Source: CAD feature listing. Evaluate the final solid. Frame: model axes, mm. Face numbers are marked on the shaded views. A direction names the side the tool comes from. Round coordinates to 2 decimals unless told otherwise and drop trailing zeros. Write each loop counter-clockwise with the first axis right and the second up, starting at its lowest first coordinate (ties: lowest second). Pieces come first, ordered by that corner, then holes.
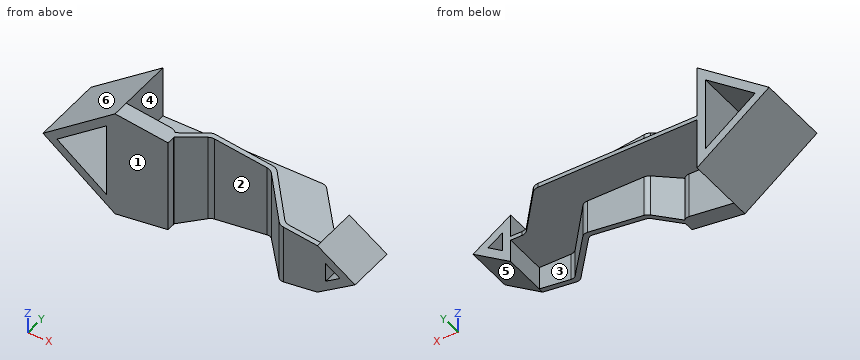
```python
from build123d import *

# Parameters (mm, degrees)
EXTRUDE_1_DEPTH             = 86
EXTRUDE_1_2_DEPTH           = 64.5
EXTRUDE_1_2_DEPTH_BACK      = 64.5
EXTRUDE_5_DEPTH             = 57.333333333
CUT_EXTRUDE_5_DEPTH         = 328.099755426
CUT_EXTRUDE_5_DEPTH_BACK    = 328.099755426
SKETCH_13_OUTSIDE_W         = 475.92
SKETCH_13_OUTSIDE_H         = 215.92
RIB_START                   = -2.5
RIB_2_DEPTH                 = 5
FILLET_1_R                  = 10
CUT_EXTRUDE_3_DEPTH         = 322.504665596
CUT_EXTRUDE_3_DEPTH_BACK    = 322.504665596
SKETCH_10_R                 = 5
CUT_EXTRUDE_4_DEPTH         = 322.504665596
CUT_EXTRUDE_4_DEPTH_BACK    = 322.504665596
SKETCH_11_R                 = 5
EXTRUDE_6_REACH             = 323.505
EXTRUDE_6_DIRECTION_2_REACH = 323.505


# Read off the part's stored shape, not the designer's step: 보강대2
with BuildPart() as part:
    # 스케치1 → Extrude 1 (new body)
    with BuildSketch(Plane(origin=(0, 0, 0), x_dir=(1, 0, 0), z_dir=(0, 1, 0))):
        Polygon((0, 64.5), (0, -64.5), (-86, 0), align=None)
        Polygon((-10, 44.5), (-69.333333333, 0), (-10, -44.5), align=None, mode=Mode.SUBTRACT)
    extrude(amount=EXTRUDE_1_DEPTH)


with BuildPart() as body_2:
    # 스케치3 → Extrude 1 2 (new, two sides: drawn at the far end of the back side and taken through both)
    with BuildSketch(Plane.XY.offset(-EXTRUDE_1_2_DEPTH_BACK)):
        Polygon((0, 0), (50, 0), (91.711375741, 35), (162.654022129, 35), (213, -25), (258, -25), (258, -19), (215.797845949, -19), (165.451868078, 41), (89.527554335, 41), (47.816178594, 6), (0, 6), align=None)
    extrude(amount=EXTRUDE_1_2_DEPTH + EXTRUDE_1_2_DEPTH_BACK)

    # 스케치13 outside → 컷-돌출5 (cut, two sides: drawn at the far end of the back side and taken through both)
    with BuildSketch(Plane(origin=(0, -19, 0), x_dir=(1, 0, 0), z_dir=(0, 1, 0)).offset(-CUT_EXTRUDE_5_DEPTH_BACK)):
        with Locations((108.5, 0)):
            Rectangle(SKETCH_13_OUTSIDE_W, SKETCH_13_OUTSIDE_H)
        Polygon((0, 64.5), (258, 30), (258, -30), (0, -64.5), align=None, mode=Mode.SUBTRACT)
    extrude(amount=CUT_EXTRUDE_5_DEPTH + CUT_EXTRUDE_5_DEPTH_BACK, mode=Mode.SUBTRACT)


with BuildPart() as body_3:
    # 스케치12 → 보스-돌출5 (new body)
    with BuildSketch(Plane.XZ.offset(25)):
        Polygon((258, 30), (258, -30), (303, 0), align=None)
        Polygon((268, 11.314829082), (284.972243623, 0), (268, -11.314829082), align=None, mode=Mode.SUBTRACT)
    extrude(amount=-EXTRUDE_5_DEPTH)


with BuildPart() as part_1:
    add(part.part)

    # Combine 1: union body 3, body 2
    add(body_3.part)
    add(body_2.part)

    # 보강대2 outline → 보강대2 (add)
    with BuildSketch(Plane.XY.offset(RIB_START)):
        Polygon((239.734972401, 32.333333333), (194.703292194, 86), (0, 86), (0, 6), (47.816178594, 6), (89.527554335, 41), (165.451868078, 41), (215.797845949, -19), (258, -19), (258, 32.333333333), align=None)
    extrude(amount=RIB_2_DEPTH)

    # 필렛1
    fillet_1_edges = [part_1.edges().sort_by_distance(p)[0] for p in [
        (194.703292194, 86, 0),
        (213, -25, 0),
        (215.797845949, -19, 19.071655649),
        (165.451868078, 41, 22.437811146),
        (89.527554335, 41, 27.514146076),
        (47.816178594, 6, 30.302988059),
        (50, 0, 0),
        (91.711375741, 35, 0),
        (162.654022129, 35, 0),
        (47.816178594, 6, -30.302988059),
        (89.527554335, 41, -27.514146076),
        (165.451868078, 41, -22.437811146),
        (215.797845949, -19, -19.071655649),
        (239.734972401, 32.333333333, 0),
    ]]
    fillet(fillet_1_edges, radius=FILLET_1_R)

    # 스케치10 → 컷-돌출3 (cut, two sides: drawn at the far end of the back side and taken through both)
    with BuildSketch(Plane.XY.offset(-CUT_EXTRUDE_3_DEPTH_BACK)):
        with Locations((158, -20)):
            Circle(SKETCH_10_R)
    extrude(amount=CUT_EXTRUDE_3_DEPTH + CUT_EXTRUDE_3_DEPTH_BACK, mode=Mode.SUBTRACT)

    # 스케치11 → 컷-돌출4 (cut, two sides: drawn at the far end of the back side and taken through both)
    with BuildSketch(Plane.XY.offset(-CUT_EXTRUDE_4_DEPTH_BACK)):
        with Locations(Location((53.25, 10, 0), (0, 0, 44.917604926))):
            Circle(SKETCH_11_R)
    extrude(amount=CUT_EXTRUDE_4_DEPTH + CUT_EXTRUDE_4_DEPTH_BACK, mode=Mode.SUBTRACT)

    # 보스-돌출6: up to this plane
    extrude_6_end = Plane(origin=(258, -25, 30), z_dir=(0.13254117731278448, 0, 0.9911774999043013))
    # 스케치8 → 보스-돌출6 (add, up to the surface)
    with BuildSketch(Plane.XY, mode=Mode.PRIVATE) as extrude_6_sk1:
        with BuildLine():
            Line((63.25, 0), (0, 0))
            Line((0, 0), (0, 20))
            Line((0, 20), (53.25, 20))
            ThreePointArc((53.25, 20), (60.321067812, 17.071067812), (63.25, 10))
            Line((63.25, 10), (63.25, 0))
        make_face()
    extrude_6_tool1 = split(extrude(extrude_6_sk1.sketch, amount=EXTRUDE_6_REACH, mode=Mode.PRIVATE), bisect_by=extrude_6_end, keep=Keep.BOTH, mode=Mode.PRIVATE)
    add(extrude_6_tool1.solids().sort_by_distance((31.117784, 9.865974, 0))[0])

    # 보스-돌출6 direction 2: up to this plane
    extrude_6_direction_2_end = Plane(origin=(0, -25, -64.5), z_dir=(0.13254117731278448, 0, -0.9911774999043013))
    # 스케치8 → 보스-돌출6 direction 2 (add, up to the surface)
    with BuildSketch(Plane.XY, mode=Mode.PRIVATE) as extrude_6_direction_2_sk1:
        with BuildLine():
            Line((63.25, 0), (0, 0))
            Line((0, 0), (0, 20))
            Line((0, 20), (53.25, 20))
            ThreePointArc((53.25, 20), (60.321067812, 17.071067812), (63.25, 10))
            Line((63.25, 10), (63.25, 0))
        make_face()
    extrude_6_direction_2_tool1 = split(extrude(extrude_6_direction_2_sk1.sketch, amount=-EXTRUDE_6_DIRECTION_2_REACH, mode=Mode.PRIVATE), bisect_by=extrude_6_direction_2_end, keep=Keep.BOTH, mode=Mode.PRIVATE)
    add(extrude_6_direction_2_tool1.solids().sort_by_distance((31.117784, 9.865974, 0))[0])


solid = part_1.part
```
Q1. Line query: line 1 (X direction, y = -6.5, z = 3); line 2 (X direction, y = 26, z = 4); line 3 (Y direction, x = 123, z = -23). Output: solid intervals per line, ascending.
Q2. Mould query, pull axis X, two halves, no side actions, for the marked faces 4, 5 and 6. Classes: pulls with the +X half, pulls with the -X half, needs draft (parallel to the pull), parting line crosses it, or undercut.
Q3. Section query C-C, the plane x = -51. Output: boundary loops of the cut face in (y, z).
Q4. Pin query (flat end, axial travel): P1, Ø12, axis at x = 10, y = 36, coming from the -Z side; P2, Ø5, axis at y = 7.5, z = -11, coming from the +X side; P3, Ø14, axis at y = 7, z = -13.5, coming from the -X side. Return the tip coordinate at first contact, or that it passes through.
Q5. Set-up query: the marked faces 1, 2 and 3. Return all of +Z, -Z, +X, -X, +Y, -Y with unobstructed straight access to the full face (end or side cutting, diameter ignored); none if empty.
Q6. Section query B-B, the plane z = 7. Give the number of separate pieces and of enclosed holes in the cut face, and give its area (3 significant figures).
Q7. Section query A-A, the plane y = 28. Output: boundary loops of the cut face in (x, z), and give its area (3 significant figures).
Filled in:
1. line 1: x = 197.48 to 205.31, 258 to 268, 280.47 to 298.5
1. line 2: x = -80.67 to -64, -10 to 0, 71.65 to 80.99, 170.21 to 178.04, 258 to 268, 278.97 to 297
1. line 3: y = 35 to 41
2. face 4: undercut
2. face 5: pulls with the +X half
2. face 6: pulls with the -X half
3. outline: (0, -26.25) - (86, -26.25) - (86, -13.75) - (0, -13.75) - close; (0, 13.75) - (86, 13.75) - (86, 26.25) - (0, 26.25) - close
4. P1: stops at z = -2.5
4. P2: stops at x = 290.25
4. P3: stops at x = -77.33
5. face 1: +Z, -Z, -X, -Y
5. face 2: +Z, -Z, -Y
5. face 3: -Z, +Y
6. separate pieces: 3
6. enclosed holes: 0
6. area: 6,540 mm2
7. outline: (-86, 0) - (0, -64.5) - (0, -2.5) - (74.03, -2.5) - (74.03, -54.6) - (83.37, -53.35) - (83.37, 53.35) - (74.03, 54.6) - (74.03, 2.5) - (0, 2.5) - (0, 64.5) - close; (168.53, -41.96) - (176.36, -40.92) - (176.36, -2.5) - (258, -2.5) - (258, -30) - (303, 0) - (258, 30) - (258, 2.5) - (176.36, 2.5) - (176.36, 40.92) - (168.53, 41.96) - close; hole (-69.33, 0) - (-10, -44.5) - (-10, 44.5) - close; hole (268, -11.31) - (284.97, 0) - (268, 11.31) - close
7. area: 6,500 mm2
